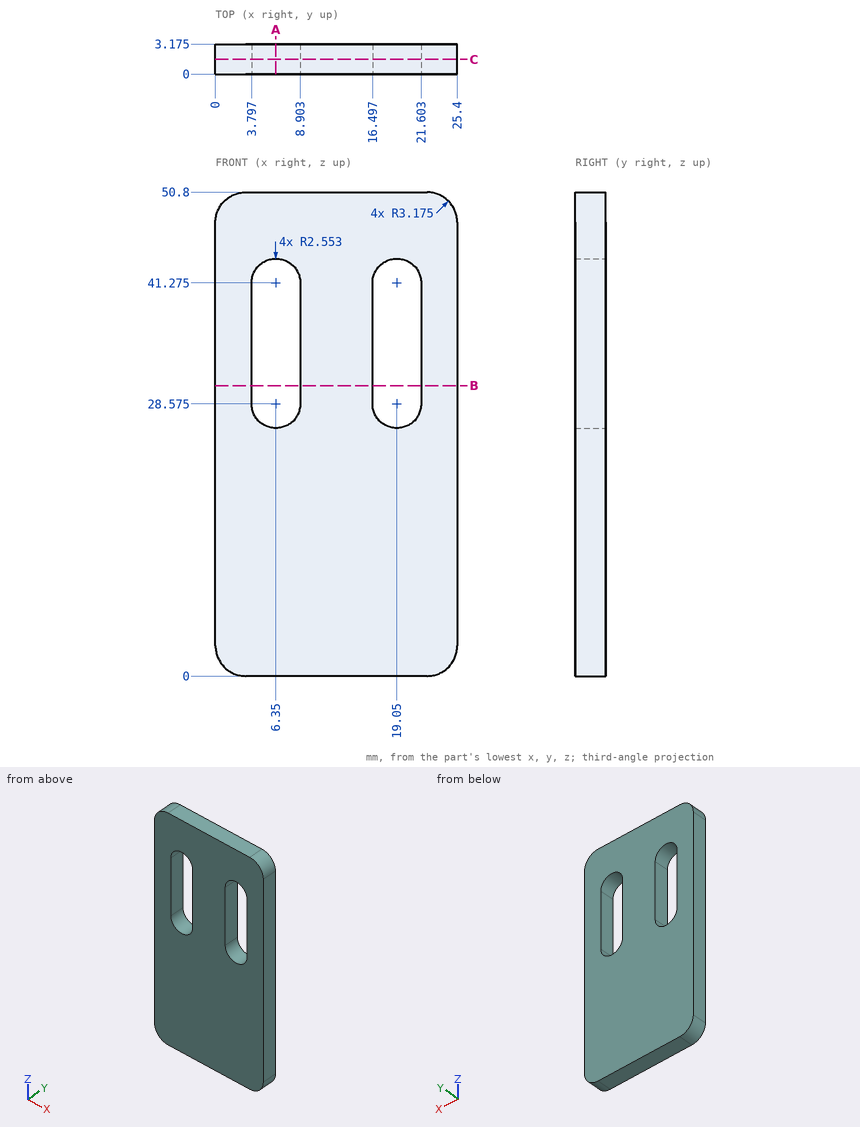
Check sheet for the drawn part. Datum: minimum x, y, z corner. Units: mm. Give positions to 0.01 mm unless a question says otherwise; leave off trailing zeros. Order: outer loops, then holes, each group sorted by start corner. A loop starts at its lowest first (then second) coordinate and runs counter-clockwise, first axis right, second up. Notation, with made-up numbers: (61.5, 48.25) - (105.5, 48.25) arc R17 ccw to (105.5, 77.25) - close; hole circle Ø4 at (32, 3.5). An arc over 180 degrees is marked (long way). Answer as a JSON object with one key per item and string values.
(1) Cross-section at A-A (x = 6.35). Record the cut outline in (y, z) (1 decimal).
Report:
{"outline": "(0, 0) - (3.2, 0) - (3.2, 26) - (0, 26) - close; (0, 43.8) - (3.2, 43.8) - (3.2, 50.8) - (0, 50.8) - close"}
(2) Cross-section at C-C (y = 1.55). State how many separate pieces and enclosed holes the cut face has, then the cut area to 3 significant figures.
Report:
{"separate pieces": "1", "enclosed holes": "2", "area": "1,110 mm^2"}
(3) Material ranges on line 1 (X direction, y = 1.5, z = 40); line 2 (Z direction, x = 4.5, y = 1.6) (1 decimal); line 3 (Z direction, x = 4, y = 2.95) (1 decimal), recorded low to high.
Report:
{"line 1": "0 to 3.8, 8.9 to 16.5, 21.6 to 25.4", "line 2": "0 to 26.8, 43 to 50.8", "line 3": "0 to 27.6, 42.3 to 50.8"}
(4) Cross-section at B-B (z = 30.5). Record the cut outline in (x, y) (1 decimal).
Report:
{"outline": "(0, 0) - (3.8, 0) - (3.8, 3.2) - (0, 3.2) - close; (8.9, 0) - (16.5, 0) - (16.5, 3.2) - (8.9, 3.2) - close; (21.6, 0) - (25.4, 0) - (25.4, 3.2) - (21.6, 3.2) - close"}
(5) Depth check by flat-ended pin: pin 1 Ø2 at (x, z) = (6.5, 34) entering from +Y. Enter the tip coordinate at first touch or a pass-through.
Report:
{"pin 1": "through"}
